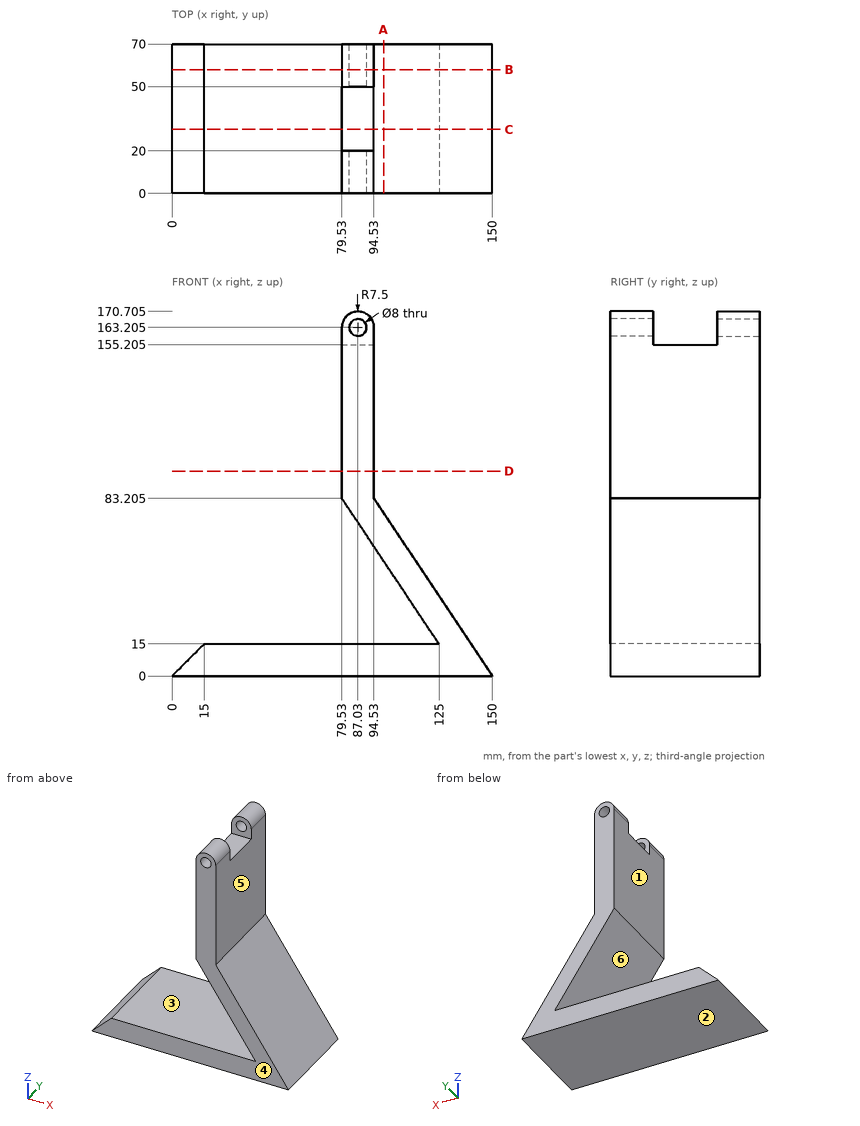
The drawing under review shows one solid part. Ordinate dimensions are in mm from its lowest x, y, z. A direction names the side the tool comes from. Give positions to 0.01 mm unless a question says otherwise; leave off trailing zeros. Loops run counter-clockwise (first coordinate to the right, second up) from the corner with the lowest first, then second, coordinate; pieces in that order, holes last. Notation, with made-up numbers: M -20.5,43.5 L -4.5,43.5 A18 ccw -4.5,53.5 Z; hole C -2,66 d5. An arc over 180 degrees is marked long. Return JSON: item names as keys, results as strings. Group by question number.
Item 1: We need section B-B (y = 58). Give the boundary of the cut face in (x, z) (3 decimals), and give its area (3 significant figures).
Item 2: We need section C-C (y = 30). Give the boundary of the cut face in (x, z) (3 decimals), and give its area (3 significant figures).
Item 3: Tool access review of the marked faces 4, 5 and 6: name each direction out of +Z, -Z, +X, -X, +Y, -Y from which nothing blocks a thin tool from reaching the whole face with its end or side.
Item 4: We need section A-A (x = 99). Give the boundary of the cut face in (y, z).
Item 5: We need section D-D (z = 96). Give the boundary of the cut face in (x, y), and give its area (3 significant figures).
Item 6: Mouldability with a two-part tool opening along Z and no side actions: class the marked faces 1, 2 and 3 as released by +Z, released by -Z, zero draft, split by the parting line, or undercut.
Item 7: Insertion check: pin 1 Ø16.5 at (x, z) = (87.5, 163.5) entering from +Y; pin 2 Ø7.5 at (x, y) = (84.5, 33.5) entering from +Z (3 decimals); pin 3 Ø8 at (y, z) = (12.5, 27) entering from -X; pin 4 Ø8 at (x, y) = (64.5, 30) entering from +Z. Each pin has a flat end and moves straight along its axis. Give the tip position at first contact, or say it passes through.
Item 8: For probe 1 along X at (y, z) = (47.5, 138.5); probe 2 along Z at (x, y) = (89, 14); probe 3 along Z at (x, y) = (68, 54), list the stretches that pass through material, from the lowest coordinate up.
Output:
{
 "1": {"outline": "M 0,0 L 150,0 L 94.53,83.205 L 94.53,163.205 A7.5 ccw 79.53,163.205 L 79.53,83.205 L 125,15 L 15,15 Z; hole C 87.03,163.205 d8", "area": "4,320 mm^2"},
 "2": {"outline": "M 0,0 L 150,0 L 94.53,83.205 L 94.53,155.205 L 79.53,155.205 L 79.53,83.205 L 125,15 L 15,15 Z", "area": "4,170 mm^2"},
 "3": {"face 4": "+Z, -Z, +X, -X, -Y", "face 5": "+Z, +X, +Y, -Y", "face 6": "-X, +Y, -Y"},
 "4": {"outline": "M 0,0 L 70,0 L 70,15 L 0,15 Z; M 0,54 L 70,54 L 70,76.5 L 0,76.5 Z"},
 "5": {"outline": "M 79.53,0 L 94.53,0 L 94.53,70 L 79.53,70 Z", "area": "1,050 mm^2"},
 "6": {"face 1": "zero draft", "face 2": "released by -Z", "face 3": "undercut"},
 "7": {"pin 1": "stops at y = 70", "pin 2": "stops at z = 155.205", "pin 3": "stops at x = 114.33", "pin 4": "stops at z = 15"},
 "8": {"probe 1": "x = 79.53 to 94.53", "probe 2": "z = 0 to 15, 69 to 159.72, 166.69 to 170.44", "probe 3": "z = 0 to 15"}
}
